Geometry check sheet. Reference: the model listing, model coordinates, mm. Face numbers are marked on the shaded views. Give positions to 0.01 mm unless a question says otherwise; leave off trailing zeros. Order: outer loops, then holes, each group sorted by start corner. A loop starts at its lowest first (then second) coordinate and runs counter-clockwise, first axis right, second up. Notation, with made-up numbers: M 0.5,-16 L 11.5,-16 A27 cw 11.5,0 Z; hole C 76.5,9 d7. An arc over 180 degrees is marked long. Answer as CSV lines item,"result". Start each with the question number.
Q1. Section check C-C, the plane x = -156.5. Record the boundary of the cut face in (y, z) (3 decimals), then the cut area to 3 significant figures.
Q2. Section check B-B, the plane z = 213. Record the boundary of the cut face in (x, y), then the cut area to 3 significant figures.
Q3. Section check A-A, the plane y = 214.5. Record the boundary of the cut face in (x, z) (3 decimals), then the cut area to 3 significant figures.
Q4. Mould release check, pull along X, two halves, no side actions. Record for the marked faces 1 and 2: +X half, -X half, draft (parallel to the pull), parting line (faces both ways), or undercut.
Q5. Go/stop test with flat-tipped pins: pin 1 (9.5 mm diameter, centred on x = -436.5, y = 177, fed in from -Z) (3 decimals); pin 2 (8 mm diameter, centred on x = 262, z = 140.5, fed in from +Y); pin 3 (21 mm diameter, centred on x = 439, z = -33, fed in from +Y). Record where each tip stops, or that it passes through.
Q6. Thickness scan on line 1 (X direction, y = 198.5, z = 402.5); line 2 (Y direction, x = -22.5, z = 150.5). Record the ranges inside material, lowest first.
```python
from build123d import *

# Parameters (mm, degrees)
F0_W     = 889
F0_H     = 895.35
F1_DEPTH = 19.05
F2_W     = 19.05
F2_H     = 895.35
F3_DEPTH = 50.8
F4_W     = 19.05
F4_H     = 88.9
F5_DEPTH = 263.525
F6_W     = 19.05
F6_H     = 88.9
F7_DEPTH = 263.525


with BuildPart() as f1:
    # F0 (on Front) → F1 (new body)
    with BuildSketch(Plane.XZ):
        Rectangle(F0_W, F0_H)
    extrude(amount=F1_DEPTH)

    # F2 (on face) → F3 (join)
    with BuildSketch(Plane(origin=(0, 0, 0), x_dir=(-1, 0, 0), z_dir=(0, 1, 0))):
        with Locations((-434.975, 0)):
            Rectangle(F2_W, F2_H)
        with Locations((434.975, 0)):
            Rectangle(F2_W, F2_H)
    extrude(amount=F3_DEPTH)

    # F4 (on face) → F5 (join)
    with BuildSketch(Plane(origin=(0, 50.8, 0), x_dir=(-1, 0, 0), z_dir=(0, 1, 0))):
        with Locations((-434.975, 403.225)):
            Rectangle(F4_W, F4_H)
    extrude(amount=F5_DEPTH)

    # F6 (on face) → F7 (join)
    with BuildSketch(Plane(origin=(0, 50.8, 0), x_dir=(-1, 0, 0), z_dir=(0, 1, 0))):
        with Locations((434.975, 403.225)):
            Rectangle(F6_W, F6_H)
    extrude(amount=F7_DEPTH)


solid = f1.part
```
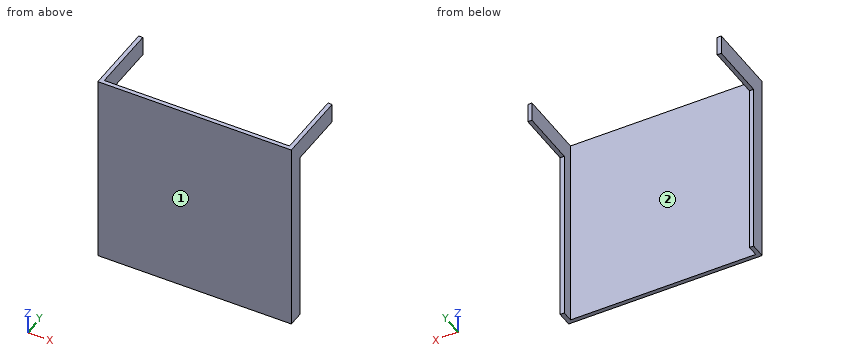
Answer block:
1,outline,"M -19.05,-447.675 L 0,-447.675 L 0,447.675 L -19.05,447.675 Z"
1,area,"17,100 mm2"
2,outline,"M -444.5,-19.05 L 444.5,-19.05 L 444.5,50.8 L 425.45,50.8 L 425.45,0 L -425.45,0 L -425.45,50.8 L -444.5,50.8 Z"
2,area,"18,900 mm2"
3,outline,"M -444.5,358.775 L -425.45,358.775 L -425.45,447.675 L -444.5,447.675 Z; M 425.45,358.775 L 444.5,358.775 L 444.5,447.675 L 425.45,447.675 Z"
3,area,"3,390 mm2"
4,face 1,"draft"
4,face 2,"undercut"
5,pin 1,"stops at z = 358.775"
5,pin 2,"stops at y = 0"
5,pin 3,"stops at y = 50.8"
6,line 1,"x = -444.5 to -425.45, 425.45 to 444.5"
6,line 2,"y = -19.05 to 0"
